Model file for the job. Use its own axes, mm. Face numbers are marked on the shaded views. Coordinates: 2 decimals unless noted, no trailing zeros. Loops run counter-clockwise (first coordinate to the right, second up) from the corner with the lowest first, then second, coordinate; pieces in that order, holes last. Notation, with made-up numbers: (27, -17) - (42, -17) arc R11 ccw to (42, -9) - close; hole circle Ø4 at (0.25, 52). An arc over 180 degrees is marked (long way). Write each question's results on one line, items separated by ' | '. Start each with the question number.
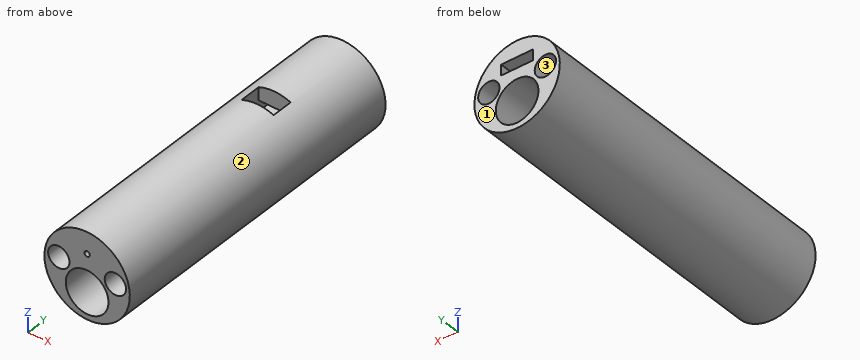
```python
from build123d import *

# Parameters (mm, degrees)
SKETCH1_R           = 4
BOSS_EXTRUDE1_DEPTH = 30
SKETCH2_W           = 3
SKETCH2_H           = 1
CUT_EXTRUDE1_DEPTH  = 10
SKETCH3_R           = 2
CUT_EXTRUDE2_DEPTH  = 30
SKETCH4_W           = 3
SKETCH4_H           = 2
CUT_EXTRUDE3_DEPTH  = 30
SKETCH5_W           = 3
SKETCH5_H           = 2
CUT_EXTRUDE5_DEPTH  = 0.5
CUT_EXTRUDE7_START  = -3
CUT_EXTRUDE7_DEPTH  = 3
CUT_EXTRUDE8_START  = -3
SKETCH8_R           = 1.25
CUT_EXTRUDE8_DEPTH  = 3
SKETCH9_R           = 0.5
CUT_EXTRUDE9_DEPTH  = 13.5
SKETCH10_R          = 0.25
CUT_EXTRUDE10_DEPTH = 30
SKETCH11_R          = 1
CUT_EXTRUDE11_DEPTH = 30


# Read off the part's stored shape, not the designer's step: Cut-Extrude7
with BuildPart() as part:
    # Sketch1 → Boss-Extrude1 (new body)
    with BuildSketch(Plane(origin=(0, 0, 0), x_dir=(1, 0, 0), z_dir=(0, 1, 0))):
        with Locations(Location((0, 0, 0), (0, 0, 270))):
            Circle(SKETCH1_R)
    extrude(amount=BOSS_EXTRUDE1_DEPTH)

    # Sketch2 → Cut-Extrude1 (cut)
    with BuildSketch(Plane(origin=(0, 30, 0), x_dir=(1, 0, 0), z_dir=(0, 1, 0))):
        with Locations((0, -2)):
            Rectangle(SKETCH2_W, SKETCH2_H)
    extrude(amount=-CUT_EXTRUDE1_DEPTH, mode=Mode.SUBTRACT)

    # Sketch3 → Cut-Extrude2 (cut)
    with BuildSketch(Plane(origin=(0, 30, 0), x_dir=(1, 0, 0), z_dir=(0, 1, 0))):
        with Locations(Location((0, 1.5, 0), (0, 0, 270))):
            Circle(SKETCH3_R)
    extrude(amount=-CUT_EXTRUDE2_DEPTH, mode=Mode.SUBTRACT)

    # Sketch4 → Cut-Extrude3 (cut)
    with BuildSketch(Plane(origin=(0, 0, 2.5), x_dir=(-1, 0, 0), z_dir=(0, 0, -1))):
        with Locations((0, 21)):
            Rectangle(SKETCH4_W, SKETCH4_H)
    extrude(amount=-CUT_EXTRUDE3_DEPTH, mode=Mode.SUBTRACT)

    # Sketch5 → Cut-Extrude5 (cut)
    with BuildSketch(Plane.XY.offset(1.5)):
        with Locations((0, 21)):
            Rectangle(SKETCH5_W, SKETCH5_H)
    extrude(amount=-CUT_EXTRUDE5_DEPTH, mode=Mode.SUBTRACT)

    # Cut-Extrude7 outline → Cut-Extrude7 (cut)
    with BuildSketch(Plane(origin=(0, 20, 0), x_dir=(1, 0, 0), z_dir=(0, 1, 0)).offset(CUT_EXTRUDE7_START)):
        with BuildLine():
            Line((1.145643924, -2.5), (1.5, -2.5))
            Line((1.5, -2.5), (1.5, -1.5))
            Line((1.5, -1.5), (1.145643924, -1.5))
            ThreePointArc((1.145643924, -1.5), (0.980237967, -1.224349609), (0.75, -1))
            Line((0.75, -1), (-0.75, -1))
            ThreePointArc((-0.75, -1), (-0.980237967, -1.224349609), (-1.145643924, -1.5))
            Line((-1.145643924, -1.5), (-1.5, -1.5))
            Line((-1.5, -1.5), (-1.5, -2.5))
            Line((-1.5, -2.5), (-1.145643924, -2.5))
            ThreePointArc((-1.145643924, -2.5), (0, -3.25), (1.145643924, -2.5))
        make_face()
    extrude(amount=CUT_EXTRUDE7_DEPTH, mode=Mode.SUBTRACT)

    # Sketch8 → Cut-Extrude8 (cut)
    with BuildSketch(Plane(origin=(0, 17, 0), x_dir=(1, 0, 0), z_dir=(0, 1, 0)).offset(CUT_EXTRUDE8_START)):
        with Locations(Location((0, -2, 0), (0, 0, 270))):
            Circle(SKETCH8_R)
    extrude(amount=CUT_EXTRUDE8_DEPTH, mode=Mode.SUBTRACT)

    # Sketch9 → Cut-Extrude9 (cut)
    with BuildSketch(Plane(origin=(0, 14, 0), x_dir=(1, 0, 0), z_dir=(0, 1, 0))):
        with Locations(Location((0, -2, 0), (0, 0, 270))):
            Circle(SKETCH9_R)
    extrude(amount=-CUT_EXTRUDE9_DEPTH, mode=Mode.SUBTRACT)

    # Sketch10 → Cut-Extrude10 (cut)
    with BuildSketch(Plane(origin=(0, 0.5, 0), x_dir=(1, 0, 0), z_dir=(0, 1, 0))):
        with Locations(Location((0, -2, 0), (0, 0, 270))):
            Circle(SKETCH10_R)
    extrude(amount=-CUT_EXTRUDE10_DEPTH, mode=Mode.SUBTRACT)

    # Sketch11 → Cut-Extrude11 (cut)
    with BuildSketch(Plane(origin=(0, 30, 0), x_dir=(1, 0, 0), z_dir=(0, 1, 0))):
        with Locations(Location((-2.65, -0.472074699, 0), (0, 0, 270))):
            Circle(SKETCH11_R)
        with Locations(Location((2.65, -0.472074699, 0), (0, 0, 270))):
            Circle(SKETCH11_R)
    extrude(amount=-CUT_EXTRUDE11_DEPTH, mode=Mode.SUBTRACT)


solid = part.part
```
Q1. Cut at B-B (z = -2). List the corners of the cut face in (x, y), and give its area (3 significant figures).
Q2. Cut at A-A (x = 3.25). List the corners of the cut face in (y, z).
Q3. Mould opens along X. For the marked faces 1, 2 and 3 say: +X half, -X half, draft (parallel to the pull), parting line (faces both ways), or undercut.
Q4. Cut at D-D (z = 0). List the corners of the cut face in (x, y).
Q5. Drill centre lines: L1, parallel to Z at x = -1, y = 15; L2, parallel to Z at x = -0.25, y = 14.5; L3, parallel to X at y = 1.75, z = 0. Where is each one in solid material? Low to high. Write a range as from..to.
Q6. Cut at C-C (y = 18.75). List the corners of the cut face in (x, z), and give its area (3 significant figures).
Q7. Pin check, flat tips, straight feed: pin 1 (1.1 mm diameter, centred on x = 0, z = 2, fed in from +Y); pin 2 (2 mm diameter, centred on y = 25.5, z = 2, fed in from -X). Stop position of each tip, or through.
Check result:
1) outline: (-3.46, 0) - (-1.94, 0) - (-1.94, 30) - (-3.46, 30) - close; (1.94, 0) - (3.46, 0) - (3.46, 30) - (1.94, 30) - close | area: 91.7 mm²
2) outline: (0, -2.33) - (30, -2.33) - (30, -0.33) - (0, -0.33) - close; (0, 1.27) - (30, 1.27) - (30, 2.33) - (0, 2.33) - close
3) face 1: draft | face 2: parting line | face 3: undercut
4) outline: (-4, 0) - (-3.53, 0) - (-3.53, 30) - (-4, 30) - close; (-1.77, 0) - (-1.32, 0) - (-1.32, 30) - (-1.77, 30) - close; (1.32, 0) - (1.77, 0) - (1.77, 30) - (1.32, 30) - close; (3.53, 0) - (4, 0) - (4, 30) - (3.53, 30) - close
5) L1: -3.87..-3.23, 0.23..1.25, 2.75..3.87 | L2: -3.99..-3.48, 0.48..0.78, 3.22..3.99 | L3: -4..-3.53, -1.77..-1.32, 1.32..1.77, 3.53..4
6) outline: circle Ø8 at (0, 0); hole circle Ø2 at (-2.65, 0.47); hole circle Ø4 at (0, -1.5); hole (-1.5, 1.5) - (-1.15, 1.5) arc R1.25 ccw to (-0.75, 1) - (0.75, 1) arc R1.25 ccw to (1.15, 1.5) - (1.5, 1.5) - (1.5, 2.5) - (1.15, 2.5) arc R1.25 ccw to (-1.15, 2.5) - (-1.5, 2.5) - close; hole circle Ø2 at (2.65, 0.47) | area: 26.2 mm²
7) pin 1: y = 30 | pin 2: x = -3.87
